from build123d import *

# Parameters (mm, degrees)
SKETCH_1_W          = 166
SKETCH_1_H          = 126
SKETCH_1_W_2        = 160
SKETCH_1_H_2        = 120
EXTRUDE_1_DEPTH     = 30
FILLET_1_R          = 5
SKETCH_2_W          = 25
SKETCH_2_H          = 10
CUT_EXTRUDE_1_DEPTH = 100
SKETCH_3_W          = 20
SKETCH_3_H          = 14
CUT_EXTRUDE_2_DEPTH = 100
SKETCH_4_W          = 120
SKETCH_4_H          = 3
CUT_EXTRUDE_3_DEPTH = 100
SKETCH_5_W          = 110
SKETCH_5_H          = 3
CUT_EXTRUDE_4_DEPTH = 100


with BuildPart() as part:
    # 草图1 → 凸台-拉伸1 (new body)
    with BuildSketch(Plane(origin=(0, 0, 0), x_dir=(1, 0, 0), z_dir=(0, 1, 0))):
        Rectangle(SKETCH_1_W, SKETCH_1_H)
        Rectangle(SKETCH_1_W_2, SKETCH_1_H_2, mode=Mode.SUBTRACT)
    extrude(amount=EXTRUDE_1_DEPTH)

    # 圆角1
    fillet_1_edges = [part.edges().sort_by_distance(p)[0] for p in [
        (83, 15, 63),
        (-83, 15, 63),
        (-83, 15, -63),
        (83, 15, -63),
    ]]
    fillet(fillet_1_edges, radius=FILLET_1_R)

    # 草图2 → 切除-拉伸1 (cut)
    with BuildSketch(Plane.XY):
        with Locations((-42.5, 18)):
            Rectangle(SKETCH_2_W, SKETCH_2_H)
    extrude(amount=CUT_EXTRUDE_1_DEPTH, mode=Mode.SUBTRACT)

    # 草图3 → 切除-拉伸2 (cut)
    with BuildSketch(Plane(origin=(0, 0, 0), x_dir=(0, 0, -1), z_dir=(1, 0, 0))):
        with Locations((-40, 15)):
            Rectangle(SKETCH_3_W, SKETCH_3_H)
    extrude(amount=CUT_EXTRUDE_2_DEPTH, mode=Mode.SUBTRACT)

    # 草图4 → 切除-拉伸3 (cut)
    with BuildSketch(Plane(origin=(0, 0, 0), x_dir=(0, 0, -1), z_dir=(1, 0, 0))):
        with Locations((0, 4)):
            Rectangle(SKETCH_4_W, SKETCH_4_H)
    extrude(amount=CUT_EXTRUDE_3_DEPTH, mode=Mode.SUBTRACT)

    # 草图5 → 切除-拉伸4 (cut)
    with BuildSketch(Plane(origin=(0, 0, 0), x_dir=(0, 0, -1), z_dir=(1, 0, 0))):
        with Locations((0, 4)):
            Rectangle(SKETCH_5_W, SKETCH_5_H)
    extrude(amount=-CUT_EXTRUDE_4_DEPTH, mode=Mode.SUBTRACT)


solid = part.part
Read the model definition and answer for the solid it produces. Units are mm, in the model's axes. A direction names the side the tool comes from. Round coordinates to 2 decimals unless told otherwise and drop trailing zeros. Write each loop counter-clockwise with the first axis right and the second up, starting at its lowest first coordinate (ties: lowest second). Pieces come first, ordered by that corner, then holes. Notation, with made-up numbers: M -21,31 L 20,31 A36 cw 20,70 Z; hole C -1.75,-32.5 d7. An arc over 180 degrees is marked long. Use a Markdown table: item, result.
1) The part is cut by section D-D (z = 48). Write down the section's boundary in (x, y), plus the area to 3 significant figures.
Answers follow:
| item | result |
|---|---|
| outline | M -83,0 L -80,0 L -80,2.5 L -83,2.5 Z; M -83,5.5 L -80,5.5 L -80,30 L -83,30 Z; M 80,0 L 83,0 L 83,2.5 L 80,2.5 Z; M 80,5.5 L 83,5.5 L 83,8 L 80,8 Z; M 80,22 L 83,22 L 83,30 L 80,30 Z |
| area | 120 mm2 |
2) The part is cut by section C-C (y = 25). Write down the section's boundary in (x, z).
Answers follow:
| item | result |
|---|---|
| outline | M -83,-58 A5 ccw -78,-63 L 78,-63 A5 ccw 83,-58 L 83,58 A5 ccw 78,63 L -78,63 A5 ccw -83,58 Z; hole M -80,-60 L 80,-60 L 80,60 L -80,60 Z |
3) The part is cut by section B-B (x = 2.5). Write down the section's boundary in (y, z).
Answers follow:
| item | result |
|---|---|
| outline | M 0,-63 L 30,-63 L 30,-60 L 0,-60 Z; M 0,60 L 30,60 L 30,63 L 0,63 Z |
4) For a pull along Z with two mould halves and no side action, classify faces 1 (the flat face through (-1, 15, 63)), 2 (the cylindrical face through (81, 15, -62)), 3 (the flat face through (-80, 15, 1)) as pulls with the +Z half, pulls with the -Z half, needs draft (parallel to the pull), parting line crosses it, or undercut.
Answers follow:
| item | result |
|---|---|
| face 1 | pulls with the +Z half |
| face 2 | pulls with the -Z half |
| face 3 | undercut |
5) A tool of negligible diameter and unlimited length cuts with its end or side. For faces 4 (the flat face through (80, 18, 1)), 5 (the flat face through (83, 18, 1)), from which of +Z, -Z, +X, -X, +Y, -Y can it reach the whole face along a straight path? Write none if from no direction.
Answers follow:
| item | result |
|---|---|
| face 4 | +Y, -Y |
| face 5 | +Z, -Z, +X, +Y, -Y |
6) Flat-ended cylindrical pins translate along their axes: pin 1 (1.5 mm diameter, centred on x = -81.5, y = 4, fed in from -Z); pin 2 (0.9 mm diameter, centred on y = 16, z = 62, fed in from -X); pin 3 (0.9 mm diameter, centred on x = 81, y = 12, fed in from -Z). Find the tip coordinate at first contact, or state that the pin passes through.
Answers follow:
| item | result |
|---|---|
| pin 1 | stops at z = -62.18 |
| pin 2 | stops at x = -81.52 |
| pin 3 | stops at z = -62.3 |
7) Straight lines are drawn through the part: line 1 along Z through (x, y) = (-37, 23.5); line 2 along X through (y, z) = (13.5, -41); line 3 along Z through (x, y) = (-48, 20.25). For each, find the intervals that lie inside material, in ascending order. Write a range as [from, to].
Answers follow:
| item | result |
|---|---|
| line 1 | z = [-63, -60], [60, 63] |
| line 2 | x = [-83, -80], [80, 83] |
| line 3 | z = [-63, -60] |
8) The part is cut by section A-A (z = -29). Write down the section's boundary in (x, y).
Answers follow:
| item | result |
|---|---|
| outline | M -83,0 L -80,0 L -80,2.5 L -83,2.5 Z; M -83,5.5 L -80,5.5 L -80,30 L -83,30 Z; M 80,0 L 83,0 L 83,2.5 L 80,2.5 Z; M 80,5.5 L 83,5.5 L 83,30 L 80,30 Z |
